```python
from build123d import *

# Parameters (mm, degrees)
F1_DEPTH = 25.4


with BuildPart() as f1:
    # F0 (on Front) → F1 (new body)
    with BuildSketch(Plane.XZ):
        Polygon((100.484227, 44.774892), (-102.714445, 44.039994), (-139.619038, 9.130239), (100.484227, 9.130239), align=None)
        Polygon((108.200631, 61.677491), (100.484227, 44.774892), (100.484227, 9.130239), (99.749338, -29.819235), (128.410263, -25.042412), (98.279542, -46.721838), (98.279542, -72.44319), (161.848029, -39.740331), (161.848029, 36.459669), align=None)
    extrude(amount=F1_DEPTH)


solid = f1.part
```
Here's how the part is built. I have some questions about the finished solid (model axes, mm). A direction names the side the tool comes from. Give positions to 0.01 mm unless a question says otherwise; leave off trailing zeros. Loops run counter-clockwise (first coordinate to the right, second up) from the corner with the lowest first, then second, coordinate; pieces in that order, holes last. Notation, with made-up numbers: (53.25, -34) -> (79.25, -34) arc R24 cw to (79.25, -4) -> close; hole circle Ø7 at (-25.75, 10). An arc over 180 degrees is marked (long way). Use one line per item in the form item = value. Start each with the question number.
1) For P1, Ø12, axis at y = -6, z = -45.5, coming from the -X side; P2, Ø1.5, axis at x = 12, y = -22.5, coming from the -Z side; P3, Ø1, axis at x = 115, y = -19, coming from the +Z side; P4, Ø3, axis at x = 97, z = -6, coming from the -Y side, each with a flat end and sliding along its axis, tell me the tip position at first contact or that it passes through.
2) Imagine slicing it at D-D (x = -33). Please give me the cut outline in (y, z).
3) Which directions (+Z, -Z, +X, -X, +Y, -Y) give clear straight access to the entire face, cutting with the end or side of a thin tool? Please do faces 1 (the face through (98.28, -13, -59)), 2 (the face through (129.62, -12.52, -56.32)).
4) Thinking about a two-plate mould opening in X: for faces 3 (the face through (43, -25.4, 10)), 4 (the face through (104.396, -12.522, 53.345)), 5 (the face through (113.6, -12.5, -35.7)), which applies, +X half, -X half, draft (parallel to the pull), parting line (faces both ways), or undercut?
5) Please list where these lines run through material, in increasing order: line 1 along X through (y, z) = (-21, 53); line 2 along X through (y, z) = (-7, -6); line 3 along Z through (x, y) = (85, -8).
6) Imagine slicing it at B-B (x = 124). Please give me the cut outline in (y, z).
7) Imagine slicing it at C-C (z = 27.5). Please give me the cut outline in (x, y).
8) Imagine slicing it at A-A (y = -6.5). Please give me the cut outline in (x, z).
Check values:
q1.P1 = 98.28
q1.P2 = 9.13
q1.P3 = 58.72
q1.P4 = through
q2.outline = (-25.4, 9.13) -> (0, 9.13) -> (0, 44.29) -> (-25.4, 44.29) -> close
q3.face_1 = -Z, -X, +Y, -Y
q3.face_2 = -Z, +X, +Y, -Y
q4.face_3 = draft
q4.face_4 = -X half
q4.face_5 = undercut
q5.line_1 = 104.24 to 126.66
q5.line_2 = 100.2 to 161.85
q5.line_3 = 9.13 to 44.72
q6.outline = (-25.4, -59.21) -> (0, -59.21) -> (0, -28.22) -> (-25.4, -28.22) -> close; (-25.4, -25.78) -> (0, -25.78) -> (0, 54.25) -> (-25.4, 54.25) -> close
q7.outline = (-120.2, -25.4) -> (161.85, -25.4) -> (161.85, 0) -> (-120.2, 0) -> close
q8.outline = (-139.62, 9.13) -> (100.48, 9.13) -> (99.75, -29.82) -> (128.41, -25.04) -> (98.28, -46.72) -> (98.28, -72.44) -> (161.85, -39.74) -> (161.85, 36.46) -> (108.2, 61.68) -> (100.48, 44.77) -> (-102.71, 44.04) -> close
